Input: dimensioned drawing with shaded views. Units: mm. Origin: part minimum x, y, z. Coordinates: 2 decimals unless noted, no trailing zeros. Order: outer loops, then holes, each group sorted by start corner. A loop starts at its lowest first (then second) coordinate and runs counter-clockwise, first axis right, second up. Notation, with made-up numbers: (55, 13) - (63, 13) arc R24 ccw to (63, 24) - close; hole circle Ø8 at (68, 67). An arc over 180 degrees is marked (long way). Use one line per item in the form item = value. Start each with the question number.
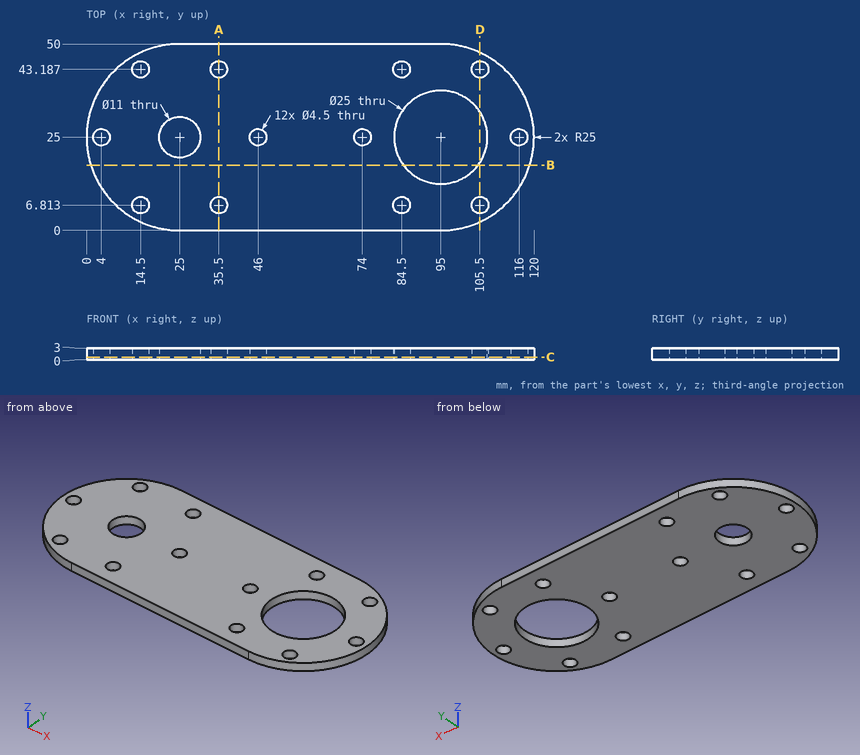
(1) Cut plane D-D on x = 105.5. Return the cut outline in (y, z).
(2) Cut plane C-C on z = 0.7. Count the separate pieces of the cut face and the enclosed holes in it, plus the area to 3 significant figures.
(3) Contact query for flat-ended pins moving along their axis: pin 1 Ø4 at (x, y) = (35.5, 43.19) entering from +Z; pin 2 Ø1 at (y, z) = (26, 1) entering from -X (1 decimal). Output: stop coordinate, or through.
(4) Material intervals for L1, parallel to Y at x = 35.5, z = 2.35; L2, parallel to X at y = 20.5, z = 1.85 (1 decimal); L3, parallel to Y at x = 46, z = 1.05, sorted ascending. Write a range as from..to.
(5) Cut plane A-A on x = 35.5. Return the cut outline in (y, z).
(6) Cut plane B-B on y = 17.5. Return the cut outline in (x, z).
Check sheet entries:
q1.outline = (2.31, 0) - (4.56, 0) - (4.56, 3) - (2.31, 3) - close; (9.06, 0) - (18.22, 0) - (18.22, 3) - (9.06, 3) - close; (31.78, 0) - (40.94, 0) - (40.94, 3) - (31.78, 3) - close; (45.44, 0) - (47.69, 0) - (47.69, 3) - (45.44, 3) - close
q2.separate_pieces = 1
q2.enclosed_holes = 14
q2.area = 4,690 mm^2
q3.pin_1 = through
q3.pin_2 = 0
q4.L1 = 0..4.56, 9.06..40.94, 45.44..50
q4.L2 = 0.4..21.8, 28.2..83.3, 106.7..119.6
q4.L3 = 0..22.75, 27.25..50
q5.outline = (0, 0) - (4.56, 0) - (4.56, 3) - (0, 3) - close; (9.06, 0) - (40.94, 0) - (40.94, 3) - (9.06, 3) - close; (45.44, 0) - (50, 0) - (50, 3) - (45.44, 3) - close
q6.outline = (1.15, 0) - (85, 0) - (85, 3) - (1.15, 3) - close; (105, 0) - (118.85, 0) - (118.85, 3) - (105, 3) - close
